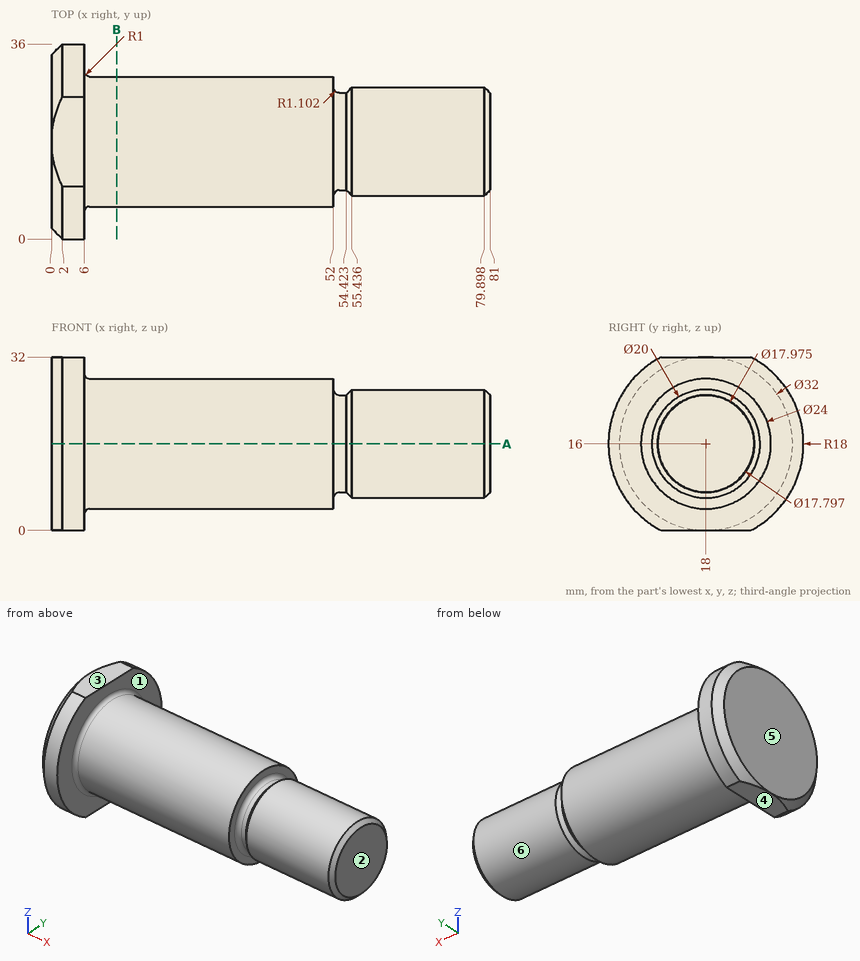
Could you check a few things on this drawing? It's one solid part, dimensions in mm from its lowest x, y, z. A direction names the side the tool comes from. Give positions to 0.01 mm unless a question says otherwise; leave off trailing zeros. Order: outer loops, then holes, each group sorted by start corner. A loop starts at its lowest first (then second) coordinate and runs counter-clockwise, first axis right, second up.
1. I need wall thicknesses on L1, parallel to X at y = 14, z = 29.5; L2, parallel to X at y = 25.5, z = 8; L3, parallel to Z at x = 4.5, y = 9.5 (1 decimal). Which ranges of each line are inside material? Lowest first, please.
Answers below:
L1: x = 0 to 6
L2: x = 0 to 52
L3: z = 0.1 to 31.9
2. Suppose I cut it at A-A (z = 16). Write out the boundary of the cut face in (x, y) (1 decimal), plus the area to 3 significant figures.
Answers below:
outline: (0, 2) - (2, 0) - (6, 0) - (6, 5) arc R1 cw to (7, 6) - (52, 6) - (52, 7.9) arc R1.1 cw to (53.1, 9) - (54.4, 9) - (55.4, 8) - (79.9, 8) - (81, 9.1) - (81, 26.9) - (79.9, 28) - (55.4, 28) - (54.4, 27) - (53.1, 27) arc R1.1 cw to (52, 28.1) - (52, 30) - (7, 30) arc R1 cw to (6, 31) - (6, 36) - (2, 36) - (0, 34) - close
area: 1,890 mm2
3. For pin 1 (10 mm diameter, centred on x = 51.5, z = 10, fed in from -Y); pin 2 (10 mm diameter, centred on y = 31.5, z = 26, fed in from +X); pin 3 (12 mm diameter, centred on x = 10, y = 11.5, fed in from +Z); pin 4 (1 mm diameter, centred on y = 25.5, z = 4, fed in from +X), each with a flat end and sliding along its axis, tell me the tip position at first contact or that it passes through.
Answers below:
pin 1: stops at y = 6.04
pin 2: stops at x = 52
pin 3: stops at z = 32
pin 4: stops at x = 6
4. Which directions (+Z, -Z, +X, -X, +Y, -Y) give clear straight access to the entire face, cutting with the end or side of a thin tool? Please do the marked faces 1 and 2.
Answers below:
face 1: +X
face 2: +Z, -Z, +X, +Y, -Y
5. Suppose I cut it at B-B (x = 12). Write out the boundary of the cut face in (y, z).
Answers below:
outline: circle Ø24 at (18, 16)
6. Thinking about a two-plate mould opening in Z: for the marked faces 3, 4, 5 and 6, which applies, +Z half, -Z half, draft (parallel to the pull), parting line (faces both ways), or undercut?
Answers below:
face 3: +Z half
face 4: -Z half
face 5: draft
face 6: parting line
